Work out the finished part from the listing and answer in its coordinate system (mm). Face numbers are marked on the shaded views. Round coordinates to 2 decimals unless told otherwise and drop trailing zeros. Loops run counter-clockwise (first coordinate to the right, second up) from the corner with the lowest first, then second, coordinate; pieces in that order, holes last. Notation, with made-up numbers: (19, 27.5) - (64, 27.5) arc R21 cw to (64, 49.5) - close; hole circle Ø8 at (56, 32). An arc over 180 degrees is marked (long way). Return JSON: item names as keys, results as strings.
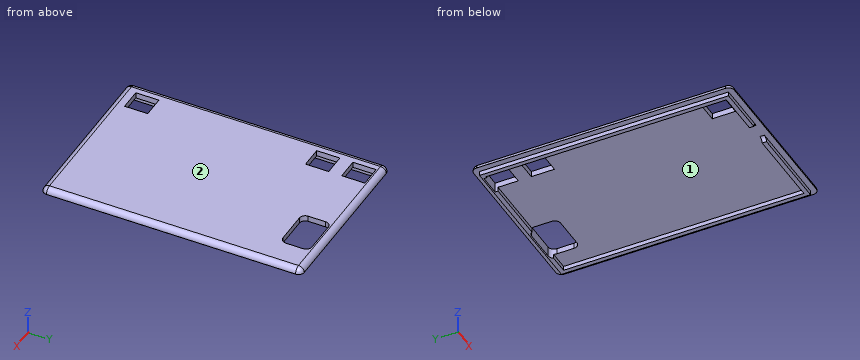
from build123d import *

# Parameters (mm, degrees)
BOX001_W             = 59
BOX001_H             = 90
BOX001_DEPTH         = 2
SKETCH003_W          = 55
SKETCH003_H          = 86
SKETCH003_W_2        = 52
SKETCH003_H_2        = 83
PAD_DEPTH            = 1.5
SKETCH002_W          = 7.5
SKETCH002_H          = 8
POCKET002_DEPTH      = 2.001
POCKET002_DEPTH_BACK = 1.501
FILLET001_R          = 1.99
POCKET003_DEPTH      = 3.501


with BuildPart() as part:
    # Box001 → Box001 (join)
    with BuildSketch(Plane.XY):
        with Locations((29.5, 45)):
            Rectangle(BOX001_W, BOX001_H)
    extrude(amount=BOX001_DEPTH)

    # Sketch003 (on Face5 of Box001) → Pad (join)
    with BuildSketch(Plane(origin=(0, 0, 0), x_dir=(1, 0, 0), z_dir=(0, 0, -1))):
        with Locations((29.5, -45)):
            Rectangle(SKETCH003_W, SKETCH003_H)
        with Locations((29.5, -45)):
            Rectangle(SKETCH003_W_2, SKETCH003_H_2, mode=Mode.SUBTRACT)
    extrude(amount=PAD_DEPTH)

    # Sketch002 (on Face5 of Box001) → Pocket002 (cut, two sides)
    with BuildSketch(Plane(origin=(0, 0, 0), x_dir=(1, 0, 0), z_dir=(0, 0, -1))) as pocket002_sk:
        with Locations((7.75, -8.5)):
            Rectangle(SKETCH002_W, SKETCH002_H)
        with Locations((7.75, -71)):
            Rectangle(SKETCH002_W, SKETCH002_H)
        with Locations((7.75, -83.5)):
            Rectangle(SKETCH002_W, SKETCH002_H)
        with BuildLine():
            Line((34, -79.5), (34, -85.5))
            ThreePointArc((34, -85.5), (34.585786, -86.914214), (36, -87.5))
            Line((36, -87.5), (47, -87.5))
            ThreePointArc((47, -87.5), (48.414214, -86.914214), (49, -85.5))
            Line((49, -85.5), (49, -79.5))
            ThreePointArc((49, -79.5), (48.414214, -78.085786), (47, -77.5))
            Line((47, -77.5), (36, -77.5))
            ThreePointArc((36, -77.5), (34.585786, -78.085786), (34, -79.5))
        make_face()
    extrude(amount=-POCKET002_DEPTH, mode=Mode.SUBTRACT)
    extrude(pocket002_sk.sketch, amount=POCKET002_DEPTH_BACK, mode=Mode.SUBTRACT)

    # Fillet001
    fillet001_edges = [part.edges().sort_by_distance(p)[0] for p in [
        (0, 45, 2),
        (29.5, 0, 2),
        (59, 45, 2),
        (29.5, 90, 2),
        (59, 0, 1),
        (0, 0, 1),
        (59, 90, 1),
        (0, 90, 1),
    ]]
    fillet(fillet001_edges, radius=FILLET001_R)

    # Sketch005 (on Face14 of Pad) → Pocket003 (cut, through all)
    with BuildSketch(Plane(origin=(0, 3.5, 0), x_dir=(-1, 0, 0), z_dir=(0, 1, 0))):
        with BuildLine():
            ThreePointArc((-26, 0), (-27.06066, -0.43934), (-27.5, -1.5))
            Line((-27.5, -1.5), (-19, -1.5))
            ThreePointArc((-19, -1.5), (-19.43934, -0.43934), (-20.5, 0))
            Line((-26, 0), (-20.5, 0))
        make_face()
    extrude(amount=-POCKET003_DEPTH, mode=Mode.SUBTRACT)


solid = part.part
1) Determine the mould class of the marked faces 1 and 2 for opening direction X: pulls with the +X half, pulls with the -X half, needs draft (parallel to the pull), parting line crosses it, or undercut.
Verdict:
{"face 1": "undercut", "face 2": "needs draft"}
2) Section D-D (z = 1.15) is taken. Give the vertices of the cut face in (x, y).
Verdict:
{"outline": "(0.36, 1.99) arc R1.63 ccw to (1.99, 0.36) - (57.01, 0.36) arc R1.63 ccw to (58.64, 1.99) - (58.64, 88.01) arc R1.63 ccw to (57.01, 89.64) - (1.99, 89.64) arc R1.63 ccw to (0.36, 88.01) - close; hole (4, 4.5) - (11.5, 4.5) - (11.5, 12.5) - (4, 12.5) - close; hole (4, 67) - (11.5, 67) - (11.5, 75) - (4, 75) - close; hole (4, 79.5) - (11.5, 79.5) - (11.5, 87.5) - (4, 87.5) - close; hole (34, 79.5) arc R2 ccw to (36, 77.5) - (47, 77.5) arc R2 ccw to (49, 79.5) - (49, 85.5) arc R2 ccw to (47, 87.5) - (36, 87.5) arc R2 ccw to (34, 85.5) - close"}
3) Flat-ended cylindrical pins translate along their axes: pin 1 (0.8 mm diameter, centred on y = 61, z = -0.5, fed in from +X); pin 2 (1.6 mm diameter, centred on y = 72, z = 1, fed in from -X); pin 3 (3 mm diameter, centred on x = 43, y = 16, fed in from -Z). Find the tip coordinate at first contact, or state that the pin passes through.
Verdict:
{"pin 1": "stops at x = 57", "pin 2": "stops at x = 0.01", "pin 3": "stops at z = 0"}
4) Find the intervals of material crossed by L1, parallel to Y at x = 6.5, z = -1.25; L2, parallel to X at y = 55, z = -1.1; L3, parallel to Y at x = 51, z = -0.4, in increasing order.
Verdict:
{"L1": "y = 2 to 3.5, 87.5 to 88", "L2": "x = 2 to 3.5, 55.5 to 57", "L3": "y = 2 to 3.5, 86.5 to 88"}
5) Section B-B (y = 83.5) is taken. Count the separate pieces of the cut face and the enclosed holes in it, and give its area (3 significant figures).
Verdict:
{"separate pieces": "3", "enclosed holes": "0", "area": "75.8 mm2"}
